```python
from build123d import *

# Parameters (mm, degrees)
BOSS_EXTRUDE1_DEPTH                            = 6.35
CSK_FOR_4_FLAT_HEAD_MACHINE_SCREW1_D           = 3.2639
CSK_FOR_4_FLAT_HEAD_MACHINE_SCREW1_CSINK_D     = 5.715
CSK_FOR_4_FLAT_HEAD_MACHINE_SCREW1_CSINK_ANGLE = 82


with BuildPart() as part:
    # Sketch1 → Boss-Extrude1 (new body)
    with BuildSketch(Plane.XY):
        Polygon((72.910979943, 164.398527709), (-102.984020057, -140.260549088), (248.805979943, -140.260549088), align=None)
    extrude(amount=BOSS_EXTRUDE1_DEPTH)

    # CSK for #4 Flat Head Machine Screw1 (through all)
    with Locations(Plane(origin=(46.660241257, 106.230914569, 6.35), x_dir=(1, 0, 0), z_dir=(0, 0, 1))):
        with Locations((0, 0), (-76.2, -131.982271537), (52.501477372, 0), (128.701477372, -131.982271537)):
            CounterSinkHole(CSK_FOR_4_FLAT_HEAD_MACHINE_SCREW1_D / 2, CSK_FOR_4_FLAT_HEAD_MACHINE_SCREW1_CSINK_D / 2, counter_sink_angle=CSK_FOR_4_FLAT_HEAD_MACHINE_SCREW1_CSINK_ANGLE)


solid = part.part
```
Input: part model. Units: mm. Frame: model coordinates. Round coordinates to 2 decimals unless told otherwise and drop trailing zeros. Write each loop counter-clockwise with the first axis right and the second up, starting at its lowest first coordinate (ties: lowest second). Pieces come first, ordered by that corner, then holes. Notation, with made-up numbers: (-22, 51) -> (30, 51) arc R27 ccw to (30, 77) -> close; hole circle Ø1 at (-34.5, 0.5). An arc over 180 degrees is marked (long way). Answer as CSV lines item,"result".
1. Section A-A (z = 2). Return the cut outline in (x, y).
Geometry says:
outline,"(-102.98, -140.26) -> (248.81, -140.26) -> (72.91, 164.4) -> close; hole circle Ø3.26 at (-29.54, -25.75); hole circle Ø3.26 at (46.66, 106.23); hole circle Ø3.26 at (99.16, 106.23); hole circle Ø3.26 at (175.36, -25.75)"
2. Contact query for flat-ended pins moving along their axis: P1, Ø1.5, axis at x = -1, z = 5.5, coming from the +Y side; P2, Ø3, axis at x = 96.5, z = 2.5, coming from the +Y side; P3, Ø1.5, axis at x = 200.5, z = 1, coming from the +Y side. Output: stop coordinate, or through.
Geometry says:
P1,"stops at y = 37.68"
P2,"stops at y = 126.14"
P3,"stops at y = -55.29"
3. Ray query, L1, parallel to Y at x = 139, z = 4.5; L2, parallel to X at y = -48.5, z = 5; L3, parallel to Y at x = 91, z = 0.5. Return the intervals inside material, ascending. Write a range as [from, to].
Geometry says:
L1,"y = [-140.26, 49.93]"
L2,"x = [-50.01, 195.83]"
L3,"y = [-140.26, 133.07]"
4. Section B-B (x = 200.5). Return the cut outline in (y, z).
Geometry says:
outline,"(-140.26, 0) -> (-56.59, 0) -> (-56.59, 6.35) -> (-140.26, 6.35) -> close"
5. Section C-C (y = -102). Return the cut outline in (x, z).
Geometry says:
outline,"(-80.89, 0) -> (226.72, 0) -> (226.72, 6.35) -> (-80.89, 6.35) -> close"
